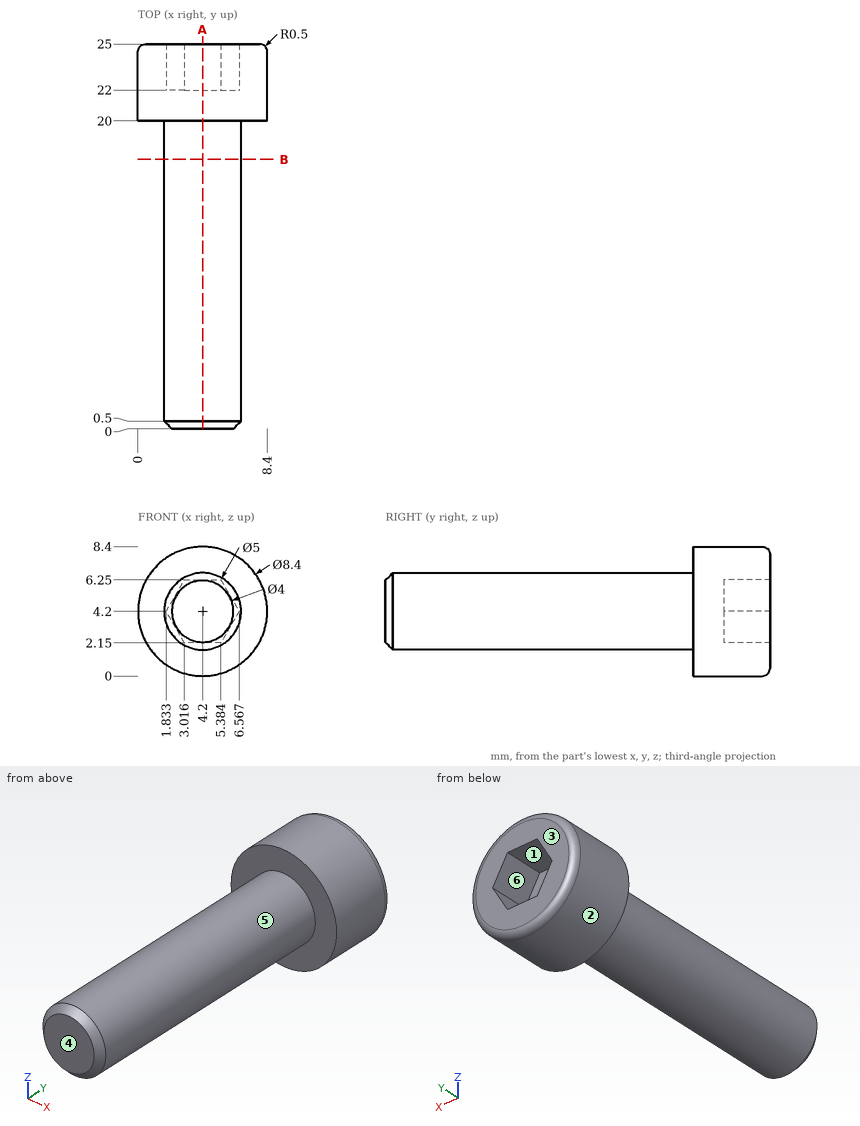
For this review, use the dimensioned drawing (mm, ordinates from the lowest corner) and the shaded views. A direction names the side the tool comes from. Coordinates: 2 decimals unless noted, no trailing zeros. Loops run counter-clockwise (first coordinate to the right, second up) from the corner with the lowest first, then second, coordinate; pieces in that order, holes last. Notation, with made-up numbers: (64.25, -16) - (89.25, -16) arc R13 cw to (89.25, 8) - close; hole circle Ø8 at (47.5, 57). An arc over 180 degrees is marked (long way). Use one line per item in the form item = value. Start each with the question number.
1) Draft analysis for pull direction Z (two halves, no side actions). For the marked faces 1, 2 and 3, state which applies: released by +Z, released by -Z, zero draft, split by the parting line, or undercut.
2) For pin 1 (2 mm diameter, centred on x = 5.5, y = 13.5, fed in from +Z); pin 2 (1.2 mm diameter, centred on x = 5, z = 3.5, fed in from +Y); pin 3 (1.5 mm diameter, centred on y = 8.5, z = 7, fed in from -X), all flat-tipped, find the tip position at first contact; note any pin that passes through.
3) Take a section at B-B (y = 17.5). State the section outline as (x, z) points.
4) Take a section at A-A (x = 4.2). State the section outline as (y, z) points.
5) To check wall thickness, follow probe 1 along Y at (x, z) = (6.5, 7); probe 2 along Z at (x, y) = (5, 7); probe 3 along X at (y, z) = (7.25, 2) (1 decimal). State the ranges of each line that lie inside material, in increasing order. Write a range as from..to.
6) For the marked faces 4, 5 and 6, list the 3-axis set-ups (+Z, -Z, +X, -X, +Y, -Y) from which the entire face can be reached by the end or side of a thin tool; tool diameter is ignored.
From the geometry:
q1.face_1 = undercut
q1.face_2 = split by the parting line
q1.face_3 = zero draft
q2.pin_1 = 6.68
q2.pin_2 = 22
q2.pin_3 = 2.77
q3.outline = circle Ø5 at (4.2, 4.2)
q4.outline = (0, 2.2) - (0.5, 1.7) - (20, 1.7) - (20, 0) - (24.5, 0) arc R0.5 ccw to (25, 0.5) - (25, 2.15) - (22, 2.15) - (22, 6.25) - (25, 6.25) - (25, 7.9) arc R0.5 ccw to (24.5, 8.4) - (20, 8.4) - (20, 6.7) - (0.5, 6.7) - (0, 6.2) - close
q5.probe_1 = 20..25
q5.probe_2 = 1.83..6.57
q5.probe_3 = 3..5.4
q6.face_4 = +Z, -Z, +X, -X, -Y
q6.face_5 = -Y
q6.face_6 = +Y
